CAD build for the part. Positions are in the model's coordinates, mm. A direction names the side the tool comes from. Round coordinates to 2 decimals unless told otherwise and drop trailing zeros. Order: outer loops, then holes, each group sorted by start corner. A loop starts at its lowest first (then second) coordinate and runs counter-clockwise, first axis right, second up. Notation, with made-up numbers: (5.25, 86) -> (12.25, 86) arc R7 cw to (12.25, 92) -> close; hole circle Ø7 at (53.5, 45.25). An arc over 180 degrees is marked (long way). Return JSON: item names as keys, results as strings. Group by question number.
Q1. Which spindle directions (+Z, -Z, +X, -X, +Y, -Y) get a long thin tool onto all of the face, cutting with end or side? Do faces 1 (the flat face through (13.3, 22, -6)), 2 (the cylindrical face through (18.73, 14.34, -2.58)). Say none if no direction does.
Q2. Cut at D-D (y = 20.5). Write the cut outline in (x, z), then the cut area to 3 significant figures.
Q3. Mould opens along Z. For faces 3 (the flat face through (10, 15, 0)), 4 (the flat face through (10, 15, -11.2)), 5 (the cylindrical face through (10.046, 26.06, -6.195)), 6 (the flat face through (8, 29.5, -6)) say: +Z half, -Z half, draft (parallel to the pull), parting line (faces both ways), or undercut.
Q4. Flat gauge pins, fed straight in: pin 1 (1.5 mm diameter, centred on x = 11.5, z = -7.5, fed in from -Y); pin 2 (1.3 mm diameter, centred on x = 4, z = -6, fed in from +Y); pin 3 (6.5 mm diameter, centred on y = 22, z = -6.5, fed in from +X). Where does each tip first touch, or does it go through?
Q5. Cut at B-B (x = 10). Write the cut outline in (y, z).
Q6. Cut at A-A (y = 13.5). Write the cut outline in (x, z).
Q7. Cut at C-C (z = -5.25). Count the separate pieces of the cut face and the enclosed holes in it, then the cut area to 3 significant figures.
Q8. Probe line 1 along Y through (x, z) = (1.05, -5.2); line 2 along Z through (x, y) = (13.75, 11); line 3 along X through (y, z) = (17.5, -4.25). List the from-to ranges inside material, lowest first.
from build123d import *

# Parameters (mm, degrees)
SKETCH6_W           = 20
SKETCH6_H           = 11.2
BOSS_EXTRUDE2_DEPTH = 29.5
SKETCH7_R           = 2.5
CUT_EXTRUDE4_DEPTH  = 38.358934674
SKETCH8_R           = 2.8
CUT_EXTRUDE5_DEPTH  = 38.358934674
SKETCH9_W           = 4.2
SKETCH9_H           = 8.2
CUT_EXTRUDE6_DEPTH  = 20
SKETCH11_R          = 1.85
CUT_EXTRUDE8_DEPTH  = 38.358934674
SKETCH12_W          = 11.2
SKETCH12_H          = 11
CUT_EXTRUDE9_DEPTH  = 6.7
CHAMFER1_SIZE       = 6.75


with BuildPart() as part:
    # Sketch6 → Boss-Extrude2 (new body)
    with BuildSketch(Plane(origin=(0, 0, 0), x_dir=(1, 0, 0), z_dir=(0, 1, 0))):
        with Locations((10, 5.6)):
            Rectangle(SKETCH6_W, SKETCH6_H)
    extrude(amount=BOSS_EXTRUDE2_DEPTH)

    # Sketch7 → Cut-Extrude4 (cut, through all)
    with BuildSketch(Plane.XY):
        with Locations((10, 5.5)):
            Circle(SKETCH7_R)
    extrude(amount=-CUT_EXTRUDE4_DEPTH, mode=Mode.SUBTRACT)

    # Sketch8 → Cut-Extrude5 (cut, through all)
    with BuildSketch(Plane.ZY):
        with Locations((-5.25, 13.5)):
            Circle(SKETCH8_R)
    extrude(amount=-CUT_EXTRUDE5_DEPTH, mode=Mode.SUBTRACT)

    # Sketch9 → Cut-Extrude6 (cut)
    with BuildSketch(Plane(origin=(0, 29.5, 0), x_dir=(1, 0, 0), z_dir=(0, 1, 0))):
        with Locations((4.6, 5.6)):
            Rectangle(SKETCH9_W, SKETCH9_H)
        with Locations((15.4, 5.6)):
            Rectangle(SKETCH9_W, SKETCH9_H)
    extrude(amount=-CUT_EXTRUDE6_DEPTH, mode=Mode.SUBTRACT)

    # Sketch11 → Cut-Extrude8 (cut, through all)
    with BuildSketch(Plane(origin=(20, 0, 0), x_dir=(0, 0, -1), z_dir=(1, 0, 0))):
        with Locations((5.2, 24.5)):
            Circle(SKETCH11_R)
    extrude(amount=-CUT_EXTRUDE8_DEPTH, mode=Mode.SUBTRACT)

    # Sketch12 → Cut-Extrude9 (cut)
    with BuildSketch(Plane(origin=(20, 0, 0), x_dir=(0, 0, -1), z_dir=(1, 0, 0))):
        with Locations((5.6, 24)):
            Rectangle(SKETCH12_W, SKETCH12_H)
    extrude(amount=-CUT_EXTRUDE9_DEPTH, mode=Mode.SUBTRACT)

    # Chamfer1
    # the kernel refuses this chamfer: 6.75 mm, written as the material it adds along each edge
    with BuildSketch(Plane(origin=(13.3, 18.5, -11.2), x_dir=(-0.027495876610586268, 0.9996219169112968, 0), z_dir=(0, 0, 1))) as chamfer1_piece_1_section:
        Polygon((CHAMFER1_SIZE * 0.999621916911, -CHAMFER1_SIZE * 0.0274958766106), (-CHAMFER1_SIZE * 0.0274958766106, -CHAMFER1_SIZE * 0.999621916911), (0, 0), align=None)
    chamfer1_piece_1 = extrude(amount=1.5, mode=Mode.PRIVATE)
    chamfer1_piece_1 = split(chamfer1_piece_1, bisect_by=Plane(origin=(17.5, 21.005794574, -10.45), z_dir=(-1, 0, 0)), keep=Keep.TOP, mode=Mode.PRIVATE)
    add(chamfer1_piece_1)
    with BuildSketch(Plane(origin=(13.3, 18.5, -11.2), x_dir=(-0.027495876610586268, 0.9996219169112968, 0), z_dir=(0, 0, 1))) as chamfer1_piece_2_section:
        Polygon((CHAMFER1_SIZE * 0.999621916911, -CHAMFER1_SIZE * 0.0274958766106), (-CHAMFER1_SIZE * 0.0274958766106, -CHAMFER1_SIZE * 0.999621916911), (0, 0), align=None)
    chamfer1_piece_2 = extrude(amount=1.5, mode=Mode.PRIVATE)
    chamfer1_piece_2 = split(chamfer1_piece_2, bisect_by=Plane(origin=(17.5, 19.207926364, -10.45), z_dir=(1, 0, 0)), keep=Keep.TOP, mode=Mode.PRIVATE)
    chamfer1_piece_2 = split(chamfer1_piece_2, bisect_by=Plane(origin=(20, 19.207926364, -10.45), z_dir=(-1, 0, 0)), keep=Keep.TOP, mode=Mode.PRIVATE)
    add(chamfer1_piece_2)
    with BuildSketch(Plane(origin=(13.3, 18.5, -11.2), x_dir=(-0.027495876610586268, 0.9996219169112968, 0), z_dir=(0, 0, 1))) as chamfer1_piece_3_section:
        Polygon((CHAMFER1_SIZE * 0.999621916911, -CHAMFER1_SIZE * 0.0274958766106), (-CHAMFER1_SIZE * 0.0274958766106, -CHAMFER1_SIZE * 0.999621916911), (0, 0), align=None)
    chamfer1_piece_3 = extrude(amount=18.858860169, mode=Mode.PRIVATE)
    chamfer1_piece_3 = split(chamfer1_piece_3, bisect_by=Plane(origin=(18.428491319, 19.207926364, -9.7), z_dir=(0, 0, 1)), keep=Keep.TOP, mode=Mode.PRIVATE)
    chamfer1_piece_3 = split(chamfer1_piece_3, bisect_by=Plane(origin=(18.428491319, 19.207926364, -1.5), z_dir=(0, 0, -1)), keep=Keep.TOP, mode=Mode.PRIVATE)
    chamfer1_piece_3 = split(chamfer1_piece_3, bisect_by=Plane(origin=(17.5, 19.207926364, -5.6), z_dir=(1, 0, 0)), keep=Keep.TOP, mode=Mode.PRIVATE)
    chamfer1_piece_3 = split(chamfer1_piece_3, bisect_by=Plane(origin=(20, 19.207926364, -5.6), z_dir=(-1, 0, 0)), keep=Keep.TOP, mode=Mode.PRIVATE)
    add(chamfer1_piece_3)
    with BuildSketch(Plane(origin=(13.3, 18.5, -11.2), x_dir=(-0.027495876610586268, 0.9996219169112968, 0), z_dir=(0, 0, 1))) as chamfer1_piece_4_section:
        Polygon((CHAMFER1_SIZE * 0.999621916911, -CHAMFER1_SIZE * 0.0274958766106), (-CHAMFER1_SIZE * 0.0274958766106, -CHAMFER1_SIZE * 0.999621916911), (0, 0), align=None)
    chamfer1_piece_4 = extrude(amount=18.858860169, mode=Mode.PRIVATE)
    chamfer1_piece_4 = split(chamfer1_piece_4, bisect_by=Plane(origin=(14.991498442, 21.005794574, 0), z_dir=(0, 0, -1)), keep=Keep.TOP, mode=Mode.PRIVATE)
    chamfer1_piece_4 = split(chamfer1_piece_4, bisect_by=Plane(origin=(14.991498442, 21.005794574, -1.5), z_dir=(0, 0, 1)), keep=Keep.TOP, mode=Mode.PRIVATE)
    chamfer1_piece_4 = split(chamfer1_piece_4, bisect_by=Plane(origin=(17.5, 21.005794574, -0.75), z_dir=(-1, 0, 0)), keep=Keep.TOP, mode=Mode.PRIVATE)
    add(chamfer1_piece_4)
    with BuildSketch(Plane(origin=(13.3, 18.5, -11.2), x_dir=(-0.027495876610586268, 0.9996219169112968, 0), z_dir=(0, 0, 1))) as chamfer1_piece_5_section:
        Polygon((CHAMFER1_SIZE * 0.999621916911, -CHAMFER1_SIZE * 0.0274958766106), (-CHAMFER1_SIZE * 0.0274958766106, -CHAMFER1_SIZE * 0.999621916911), (0, 0), align=None)
    chamfer1_piece_5 = extrude(amount=18.858860169, mode=Mode.PRIVATE)
    chamfer1_piece_5 = split(chamfer1_piece_5, bisect_by=Plane(origin=(18.428491319, 19.207926364, 0), z_dir=(0, 0, -1)), keep=Keep.TOP, mode=Mode.PRIVATE)
    chamfer1_piece_5 = split(chamfer1_piece_5, bisect_by=Plane(origin=(18.428491319, 19.207926364, -1.5), z_dir=(0, 0, 1)), keep=Keep.TOP, mode=Mode.PRIVATE)
    chamfer1_piece_5 = split(chamfer1_piece_5, bisect_by=Plane(origin=(17.5, 19.207926364, -0.75), z_dir=(1, 0, 0)), keep=Keep.TOP, mode=Mode.PRIVATE)
    chamfer1_piece_5 = split(chamfer1_piece_5, bisect_by=Plane(origin=(20, 19.207926364, -0.75), z_dir=(-1, 0, 0)), keep=Keep.TOP, mode=Mode.PRIVATE)
    add(chamfer1_piece_5)


solid = part.part
Solution:
{
 "1": {"face 1": "+Y", "face 2": "+X, -X"},
 "2": {"outline": "(0, -11.2) -> (18.05, -11.2) -> (18.05, 0) -> (0, 0) -> close; hole (2.5, -9.7) -> (6.7, -9.7) -> (6.7, -1.5) -> (2.5, -1.5) -> close; hole (13.3, -9.7) -> (17.5, -9.7) -> (17.5, -1.5) -> (13.3, -1.5) -> close", "area": "133 mm²"},
 "3": {"face 3": "+Z half", "face 4": "-Z half", "face 5": "undercut", "face 6": "draft"},
 "4": {"pin 1": "stops at y = 0", "pin 2": "stops at y = 9.5", "pin 3": "stops at x = 19.8"},
 "5": {"outline": "(0, -11.2) -> (3, -11.2) -> (3, 0) -> (0, 0) -> close; (8, -11.2) -> (29.5, -11.2) -> (29.5, 0) -> (8, 0) -> close; hole circle Ø5.6 at (13.5, -5.25); hole circle Ø3.7 at (24.5, -5.2)"},
 "6": {"outline": "(0, -11.2) -> (20, -11.2) -> (20, -8.05) -> (17.5, -8.05) -> (17.5, -9.7) -> (13.3, -9.7) -> (13.3, -8.05) -> (6.7, -8.05) -> (6.7, -9.7) -> (2.5, -9.7) -> (2.5, -8.05) -> (0, -8.05) -> close; (0, -2.45) -> (2.5, -2.45) -> (2.5, -1.5) -> (6.7, -1.5) -> (6.7, -2.45) -> (13.3, -2.45) -> (13.3, -1.5) -> (17.5, -1.5) -> (17.5, -2.45) -> (20, -2.45) -> (20, 0) -> (0, 0) -> close"},
 "7": {"separate pieces": "6", "enclosed holes": "1", "area": "279 mm²"},
 "8": {"line 1": "y = 0 to 10.7, 16.3 to 22.65, 26.35 to 29.5", "line 2": "z = -11.2 to -9.7, -1.5 to 0", "line 3": "x = 0 to 2.5, 6.7 to 13.3, 17.5 to 20"}
}
